Verification items for the finished model (mm, model axes). Face numbers are marked on the shaded views. A direction names the side the tool comes from. Give positions to 0.01 mm unless a question says otherwise; leave off trailing zeros. Order: outer loops, then holes, each group sorted by start corner. A loop starts at its lowest first (then second) coordinate and runs counter-clockwise, first axis right, second up. Notation, with made-up numbers: (62, 16.5) - (88, 16.5) arc R23 cw to (88, 36.5) - close; hole circle Ø7 at (41, 67). An arc over 180 degrees is marked (long way). Answer as a JSON object with one key per item and string values. Group by question number.
(1) Section check D-D (x = -3). Record the boundary of the cut face in (y, z).
(2) Thickness scan on line 1 (X direction, y = -42, z = -9); line 2 (X direction, y = -43.2, z = 0); line 3 (Z direction, x = 1.5, y = -12.5). Record the ranges inside material, lowest first.
(3) Access from +Z, -Z, +X, -X, +Y, -Y to the whole of each face (thin tool, end or side, straight path). Record for the marked faces 1 and 2.
(4) Depth check by flat-ended pin: pin 1 Ø5 at (x, y) = (0, 0) entering from +Z; pin 2 Ø3.5 at (y, z) = (-5.5, 20.5) entering from +X; pin 3 Ø1.5 at (y, z) = (-2.5, 21) entering from -X; pin 4 Ø14 at (x, z) = (-4, 3) entering from +Y. Enter the tip coordinate at first touch or a pass-through.
(5) Section check B-B (y = -5). Record the boundary of the cut face in (x, z).
(6) Section check C-C (z = -4). Record the boundary of the cut face in (x, y), then the cut area to 3 significant figures.
(7) Section check A-A (z = 9). Record the boundary of the cut face in (x, y).
(8) Mould release check, pull along Z, two halves, no side actions. Record for the marked faces 3, 4 and 5: +Z half, -Z half, draft (parallel to the pull), parting line (faces both ways), or undercut.
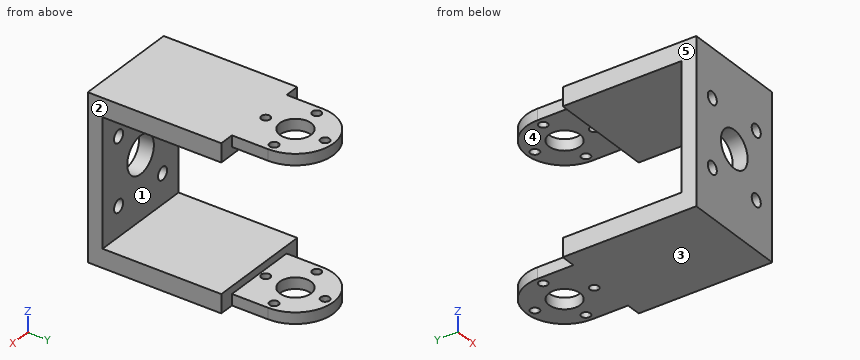
```python
from build123d import *

# Parameters (mm, degrees)
BOSS_EXTRUDE1_DEPTH      = 22
BOSS_EXTRUDE1_DEPTH_BACK = 22
SKETCH2_W                = 38
SKETCH2_H                = 20
CUT_EXTRUDE1_DEPTH       = 105.423416914
SKETCH3_W                = 7
SKETCH3_H                = 44
BOSS_EXTRUDE2_DEPTH      = 36
SKETCH5_W                = 34
SKETCH5_H                = 50
CUT_EXTRUDE3_DEPTH       = 109.047443283
SKETCH6_W                = 20.5
SKETCH6_H                = 54.25
CUT_EXTRUDE4_DEPTH       = 111.605436123
SKETCH20_W               = 28.5
SKETCH20_H               = 34
SKETCH20_R               = 1.7
SKETCH20_R_2             = 5
BOSS_EXTRUDE5_DEPTH      = 4
SKETCH21_W               = 3
SKETCH21_H               = 36
CUT_EXTRUDE12_DEPTH      = 66.777085676


with BuildPart() as part:
    # Sketch1 → Boss-Extrude1 (new, two sides: drawn at the far end of the back side and taken through both)
    with BuildSketch(Plane.XY.offset(-BOSS_EXTRUDE1_DEPTH_BACK)):
        with BuildLine():
            Line((10.25, -60), (10.25, 0))
            ThreePointArc((10.25, 0), (0, -10.25), (-10.25, 0))
            Line((-10.25, 0), (-10.25, -60))
            Line((-10.25, -60), (-10.25, -100))
            Line((-10.25, -100), (10.25, -100))
            Line((10.25, -100), (10.25, -60))
        make_face()
        with BuildLine():
            Line((10.25, 0), (9.2, 0))
            ThreePointArc((9.2, 0), (8.816088231, -0.879772698), (7.91, -1.196620241))
            ThreePointArc((7.91, -1.196620241), (5.656854249, -5.656854249), (1.196620241, -7.91))
            ThreePointArc((1.196620241, -7.91), (1.199154762, -7.954968281), (1.2, -8))
            ThreePointArc((1.2, -8), (-0.045031719, -9.199154762), (-1.196620241, -7.91))
            ThreePointArc((-1.196620241, -7.91), (-5.656854249, -5.656854249), (-7.91, -1.196620241))
            ThreePointArc((-7.91, -1.196620241), (-8.816088231, -0.879772698), (-9.2, 0))
            Line((-9.2, 0), (-10.25, 0))
            ThreePointArc((-10.25, 0), (0, -10.25), (10.25, 0))
        make_face()
        with BuildLine():
            ThreePointArc((7.91, -1.196620241), (7.120227302, -0.816088231), (6.8, 0))
            Line((6.8, 0), (4.2, 0))
            ThreePointArc((4.2, 0), (0, -4.2), (-4.2, 0))
            Line((-4.2, 0), (-6.8, 0))
            ThreePointArc((-6.8, 0), (-7.120227302, -0.816088231), (-7.91, -1.196620241))
            ThreePointArc((-7.91, -1.196620241), (-5.656854249, -5.656854249), (-1.196620241, -7.91))
            ThreePointArc((-1.196620241, -7.91), (0, -6.8), (1.196620241, -7.91))
            ThreePointArc((1.196620241, -7.91), (5.656854249, -5.656854249), (7.91, -1.196620241))
        make_face()
        with BuildLine():
            Line((4.2, 0), (6.8, 0))
            ThreePointArc((6.8, 0), (7.120227302, 0.816088231), (7.91, 1.196620241))
            ThreePointArc((7.91, 1.196620241), (5.656854249, 5.656854249), (1.196620241, 7.91))
            ThreePointArc((1.196620241, 7.91), (0, 6.8), (-1.196620241, 7.91))
            ThreePointArc((-1.196620241, 7.91), (-5.656854249, 5.656854249), (-7.91, 1.196620241))
            ThreePointArc((-7.91, 1.196620241), (-7.120227302, 0.816088231), (-6.8, 0))
            Line((-6.8, 0), (-4.2, 0))
            ThreePointArc((-4.2, 0), (0, 4.2), (4.2, 0))
        make_face()
        with BuildLine():
            ThreePointArc((7.91, 1.196620241), (8.816088231, 0.879772698), (9.2, 0))
            Line((9.2, 0), (10.25, 0))
            ThreePointArc((10.25, 0), (0, 10.25), (-10.25, 0))
            Line((-10.25, 0), (-9.2, 0))
            ThreePointArc((-9.2, 0), (-8.816088231, 0.879772698), (-7.91, 1.196620241))
            ThreePointArc((-7.91, 1.196620241), (-5.656854249, 5.656854249), (-1.196620241, 7.91))
            ThreePointArc((-1.196620241, 7.91), (-0.045031719, 9.199154762), (1.2, 8))
            ThreePointArc((1.2, 8), (1.199154762, 7.954968281), (1.196620241, 7.91))
            ThreePointArc((1.196620241, 7.91), (5.656854249, 5.656854249), (7.91, 1.196620241))
        make_face()
    extrude(amount=BOSS_EXTRUDE1_DEPTH + BOSS_EXTRUDE1_DEPTH_BACK)

    # Sketch2 → Cut-Extrude1 (cut, through all)
    with BuildSketch(Plane.ZY.offset(10.25)):
        with Locations((0, 0.25)):
            Rectangle(SKETCH2_W, SKETCH2_H)
    extrude(amount=-CUT_EXTRUDE1_DEPTH, mode=Mode.SUBTRACT)

    # Sketch3 → Boss-Extrude2 (add)
    with BuildSketch(Plane(origin=(0, -9.75, 0), x_dir=(1, 0, 0), z_dir=(0, 1, 0))):
        with Locations((-13.75, 0)):
            Rectangle(SKETCH3_W, SKETCH3_H)
        with Locations((13.75, 0)):
            Rectangle(SKETCH3_W, SKETCH3_H)
    extrude(amount=-BOSS_EXTRUDE2_DEPTH)

    # Sketch5 → Cut-Extrude3 (cut, through all)
    with BuildSketch(Plane.ZY.offset(17.25)):
        with Locations((0, -34.75)):
            Rectangle(SKETCH5_W, SKETCH5_H)
    extrude(amount=-CUT_EXTRUDE3_DEPTH, mode=Mode.SUBTRACT)

    # Sketch6 → Cut-Extrude4 (cut, through all)
    with BuildSketch(Plane.XY.offset(22)):
        with Locations((0, -72.875)):
            Rectangle(SKETCH6_W, SKETCH6_H)
    extrude(amount=-CUT_EXTRUDE4_DEPTH, mode=Mode.SUBTRACT)


with BuildPart() as cut_extrude4_piece_1:
    # of the separate pieces the step leaves, piece 1, a body of its own (cut_extrude4_pieces)
    add(part.part.solids().sort_by_distance((10.25, 0, -22))[0])



with BuildPart() as cut_extrude4_piece_2:
    # of the separate pieces the step leaves, piece 2, a body of its own (cut_extrude4_pieces)
    add(part.part.solids().sort_by_distance((17.25, -45.75, 22))[0])


with BuildPart() as cut_extrude4_piece_1_1:
    add(cut_extrude4_piece_1.part)

    add(cut_extrude4_piece_2.part)  # Boss-Extrude5 merges Cut-Extrude4 piece 2
    # Sketch20 → Boss-Extrude5 (add)
    with BuildSketch(Plane.XZ.offset(45.75)):
        Rectangle(SKETCH20_W, SKETCH20_H)
        with Locations(Location((-8.25, -9, 0), (0, 0, 270))):
            Circle(SKETCH20_R, mode=Mode.SUBTRACT)
        with Locations(Location((8.25, -9, 0), (0, 0, 270))):
            Circle(SKETCH20_R, mode=Mode.SUBTRACT)
        with Locations(Location((-8.25, 9, 0), (0, 0, 270))):
            Circle(SKETCH20_R, mode=Mode.SUBTRACT)
        with Locations(Location((0, 0, 0), (0, 0, 270))):
            Circle(SKETCH20_R_2, mode=Mode.SUBTRACT)
        with Locations(Location((8.25, 9, 0), (0, 0, 270))):
            Circle(SKETCH20_R, mode=Mode.SUBTRACT)
    extrude(amount=-BOSS_EXTRUDE5_DEPTH)

    # Sketch21 → Cut-Extrude12 (cut, through all)
    with BuildSketch(Plane(origin=(0, 0, -22), x_dir=(-1, 0, 0), z_dir=(0, 0, -1))):
        with Locations((-15.75, -27.75)):
            Rectangle(SKETCH21_W, SKETCH21_H)
        with Locations((15.75, -27.75)):
            Rectangle(SKETCH21_W, SKETCH21_H)
    extrude(amount=-CUT_EXTRUDE12_DEPTH, mode=Mode.SUBTRACT)


solid = cut_extrude4_piece_1_1.part
```
Solutions:
{
 "1": {"outline": "(-45.75, -22) - (-2.94, -22) - (-2.94, -19) - (-9.75, -19) - (-9.75, -17) - (-41.75, -17) - (-41.75, -4) - (-45.75, -4) - close; (-45.75, 4) - (-41.75, 4) - (-41.75, 17) - (-9.75, 17) - (-9.75, 19) - (-2.94, 19) - (-2.94, 22) - (-45.75, 22) - close; (2.94, -22) - (9.8, -22) - (9.8, -19) - (2.94, -19) - close; (2.94, 19) - (9.8, 19) - (9.8, 22) - (2.94, 22) - close"},
 "2": {"line 1": "x = -14.25 to -9.95, -6.55 to 6.55, 9.95 to 14.25", "line 2": "x = -14.25 to -5, 5 to 14.25", "line 3": "z = -22 to -17, 17 to 22"},
 "3": {"face 1": "+X, -X, +Y", "face 2": "+Z, -Z, +X, +Y, -Y"},
 "4": {"pin 1": "passes through", "pin 2": "stops at x = 10.25", "pin 3": "stops at x = -10.25", "pin 4": "stops at y = -41.75"},
 "5": {"outline": "(-10.25, -22) - (10.25, -22) - (10.25, -19) - (-10.25, -19) - close; (-10.25, 19) - (10.25, 19) - (10.25, 22) - (-10.25, 22) - close"},
 "6": {"outline": "(-14.25, -45.75) - (-3, -45.75) - (-3, -41.75) - (-14.25, -41.75) - close; (3, -45.75) - (14.25, -45.75) - (14.25, -41.75) - (3, -41.75) - close", "area": "90.0 mm2"},
 "7": {"outline": "(-14.25, -45.75) - (-9.95, -45.75) - (-9.95, -41.75) - (-14.25, -41.75) - close; (-6.55, -45.75) - (6.55, -45.75) - (6.55, -41.75) - (-6.55, -41.75) - close; (9.95, -45.75) - (14.25, -45.75) - (14.25, -41.75) - (9.95, -41.75) - close"},
 "8": {"face 3": "-Z half", "face 4": "undercut", "face 5": "draft"}
}
